Here's how the part is built. I have some questions about the finished solid (model axes, mm). Coordinates: 2 decimals unless noted, no trailing zeros. Write each loop counter-clockwise with the first axis right and the second up, starting at its lowest first coordinate (ties: lowest second). Pieces come first, ordered by that corner, then holes.
(1) For pin 1 Ø5 at (x, z) = (15.5, 17.5) entering from +Y; pin 2 Ø20 at (x, y) = (27.36, 21.82) entering from -Z; pin 3 Ø4 at (y, z) = (3.5, 19.5) entering from -X; pin 4 Ø12 at (x, z) = (-29.5, 44) entering from +Y, each with a flat end and sliding along its axis, tell me the tip position at first contact or that it passes through.
(2) Imagine slicing it at B-B, the plane y = -4.5. List the corners of the cut face in (x, z) for me, plus the area to 3 significant figures.
(3) Imagine slicing it at C-C, the plane x = 32. List the corners of the cut face in (y, z) for me, plus the area to 3 significant figures.
(4) Thinking about a two-plate mould opening in Y: for faces 1 (the cylindrical face through (-2.71, 22.797, 25.35)), 2 (the cylindrical face through (47.69, 15.02, 24.65)), 3 (the flat face through (-1, 1, 0)), which applies, released by +Y, released by -Y, zero draft, split by the parting line, or undercut?
(5) Please list where these lines run through material, in increasing order: probe 1 along Y at (x, z) = (-4, 28); probe 2 along Y at (x, z) = (38, 22); probe 3 along Y at (x, z) = (-24, 44).
(6) Imagine slicing it at D-D, the plane z = 22. List the corners of the cut face in (x, y) for me, plus the area to 3 significant figures.
(7) Imagine slicing it at A-A, the plane x = 0. List the corners of the cut face in (y, z) for me.
```python
from build123d import *

# Parameters (mm, degrees)
F0_R     = 50
F1_DEPTH = 50
F2_R     = 12.5
F3_DEPTH = 50


with BuildPart() as f1:
    # F0 (on Top) → F1 (new body)
    with BuildSketch(Plane.XY):
        Circle(F0_R)
    extrude(amount=F1_DEPTH)

    # F2 (on face) → F3 (cut, through all)
    with BuildSketch(Plane.XY.offset(50)):
        with Locations((-15.185931, -31.53391)):
            Circle(F2_R)
        with Locations((15.185931, -31.53391)):
            Circle(F2_R)
        with Locations((34.122477, -7.788233)):
            Circle(F2_R)
        with Locations((27.364102, 21.822143)):
            Circle(F2_R)
        with Locations((0, 35)):
            Circle(F2_R)
        with Locations((-27.364102, 21.822143)):
            Circle(F2_R)
        with Locations((-34.122477, -7.788233)):
            Circle(F2_R)
    extrude(amount=-F3_DEPTH, mode=Mode.SUBTRACT)


solid = f1.part
```
Recorded:
1. pin 1: stops at y = 48.28
1. pin 2: passes through
1. pin 3: stops at x = -49.98
1. pin 4: stops at y = 44.13
2. outline: (-49.8, 0) - (-46.18, 0) - (-46.18, 50) - (-49.8, 50) - close; (-22.06, 0) - (22.06, 0) - (22.06, 50) - (-22.06, 50) - close; (46.18, 0) - (49.8, 0) - (49.8, 50) - (46.18, 50) - close
2. area: 2,570 mm2
3. outline: (-38.42, 0) - (-20.11, 0) - (-20.11, 50) - (-38.42, 50) - close; (4.53, 0) - (10.21, 0) - (10.21, 50) - (4.53, 50) - close; (33.43, 0) - (38.42, 0) - (38.42, 50) - (33.43, 50) - close
3. area: 1,450 mm2
4. face 1: undercut
4. face 2: split by the parting line
4. face 3: zero draft
5. probe 1: y = -49.84 to -37.11, -25.95 to 23.16, 46.84 to 49.84
5. probe 2: y = -32.5 to -19.67, 4.1 to 15.25, 28.39 to 32.5
5. probe 3: y = -43.86 to -40.4, -22.67 to -15.12, -0.45 to 9.78, 33.86 to 43.86
6. outline: circle Ø100 at (0, 0); hole circle Ø25 at (-34.12, -7.79); hole circle Ø25 at (-27.36, 21.82); hole circle Ø25 at (-15.19, -31.53); hole circle Ø25 at (0, 35); hole circle Ø25 at (15.19, -31.53); hole circle Ø25 at (27.36, 21.82); hole circle Ø25 at (34.12, -7.79)
6. area: 4,420 mm2
7. outline: (-50, 0) - (22.5, 0) - (22.5, 50) - (-50, 50) - close; (47.5, 0) - (50, 0) - (50, 50) - (47.5, 50) - close
